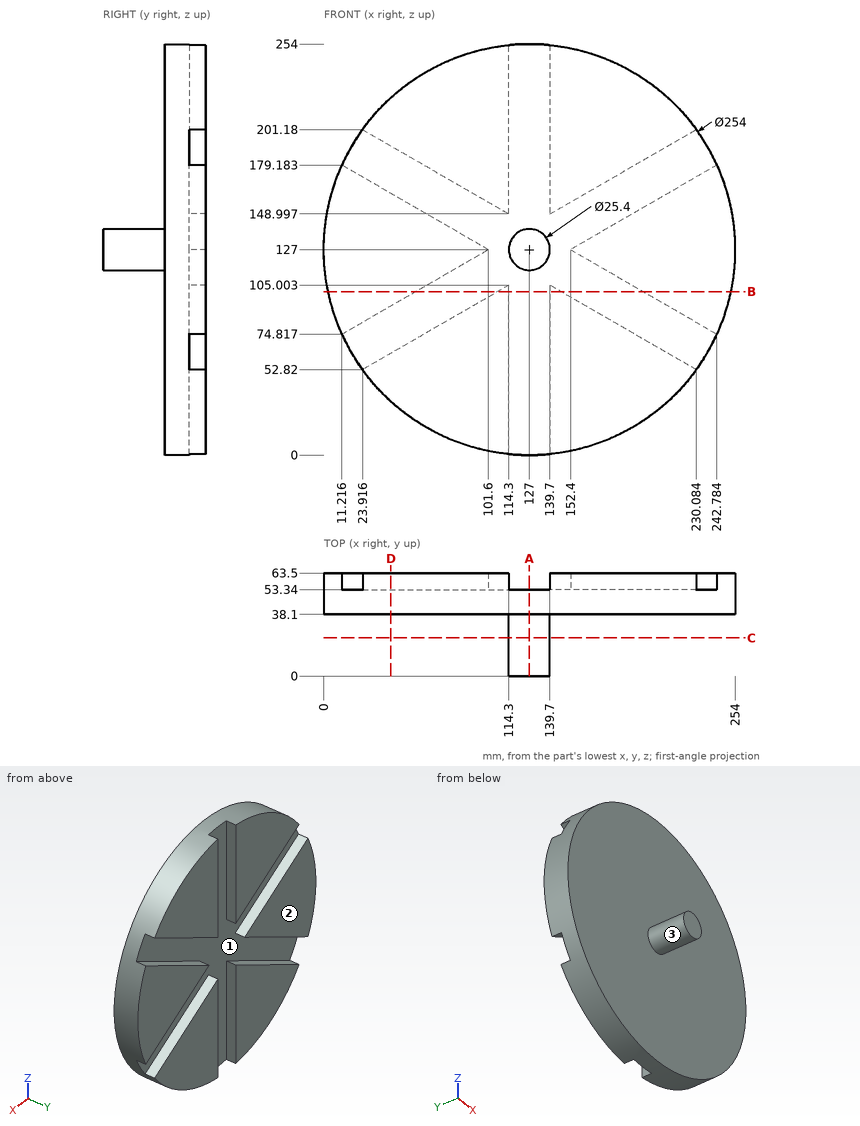
Print and shaded views of the part. All mm, measured from the part's lowest x, y and z. Round coordinates to 2 decimals unless told otherwise and drop trailing zeros. Write each loop counter-clockwise with the first axis right and the second up, starting at its lowest first coordinate (ties: lowest second). Pieces come first, ordered by that corner, then holes. Notation, with made-up numbers: (-3, 7) -> (21, 7) arc R36 ccw to (21, 46) -> close; hole circle Ø10 at (-15.5, 8). An arc over 180 degrees is marked (long way). Write item = value, one per line.
(1) Flat gauge pins, fed straight in: pin 1 (12 mm diameter, centred on y = 31, z = 162.5, fed in from +X) (3 decimals); pin 2 (2 mm diameter, centred on y = 40, z = 113, fed in from +X); pin 3 (11 mm diameter, centred on y = 59.5, z = 71.5, fed in from +X); pin 4 (1.5 mm diameter, centred on x = 161, y = 49.5, fed in from -Z). Where does each tip first touch, or does it go through?
Answer:
pin_1 = through
pin_2 = 253.33
pin_3 = 243.74
pin_4 = 4.43
(2) Band-saw the part on D-D (x = 41.5). Give the cut face in (y, z), then the cut area to 3 significant figures.
Answer:
outline = (38.1, 33.09) -> (63.5, 33.09) -> (63.5, 62.97) -> (53.34, 62.97) -> (53.34, 92.3) -> (63.5, 92.3) -> (63.5, 161.7) -> (53.34, 161.7) -> (53.34, 191.03) -> (63.5, 191.03) -> (63.5, 220.91) -> (38.1, 220.91) -> close
area = 4,170 mm2
(3) Band-saw the part on C-C (y = 23.5). Give the cut face in (x, z).
Answer:
outline = circle Ø25.4 at (127, 127)
(4) Probe L1, parallel to Z at x = 33, y = 54 (1 decimal); L2, parallel to Y at x = 233, z = 123; L3, parallel to Y at x = 139.5, z = 189. List the from-to ranges inside material, lowest first.
Answer:
L1 = 41.6 to 58.1, 87.4 to 166.6, 195.9 to 212.4
L2 = 38.1 to 63.5
L3 = 38.1 to 53.34
(5) Band-saw the part on B-B (z = 101). Give the cut face in (x, y).
Answer:
outline = (2.69, 38.1) -> (251.31, 38.1) -> (251.31, 63.5) -> (197.43, 63.5) -> (197.43, 53.34) -> (146.63, 53.34) -> (146.63, 63.5) -> (139.7, 63.5) -> (139.7, 53.34) -> (114.3, 53.34) -> (114.3, 63.5) -> (107.37, 63.5) -> (107.37, 53.34) -> (56.57, 53.34) -> (56.57, 63.5) -> (2.69, 63.5) -> close
(6) Two-plate mould, pull along X, no slides. Class the marked faces 1, 2 and 3: pulls with the +X half, pulls with the -X half, needs draft (parallel to the pull), parting line crosses it, or undercut.
Answer:
face_1 = undercut
face_2 = needs draft
face_3 = parting line crosses it
(7) Band-saw the part on A-A (x = 127). Give the cut face in (y, z), then the cut area to 3 significant figures.
Answer:
outline = (0, 114.3) -> (38.1, 114.3) -> (38.1, 0) -> (53.34, 0) -> (53.34, 254) -> (38.1, 254) -> (38.1, 139.7) -> (0, 139.7) -> close
area = 4,840 mm2
